Part model, mm, in its own coordinate system. Face numbers are marked on the shaded views. Round coordinates to 2 decimals unless told otherwise and drop trailing zeros. Write each loop counter-clockwise with the first axis right and the second up, starting at its lowest first coordinate (ties: lowest second). Pieces come first, ordered by that corner, then holes. Notation, with made-up numbers: M -10,14 L 9,14 A7 cw 9,27 Z; hole C 64,15 d6. An arc over 180 degrees is marked long. One line per question, with ' | ' between items. Start each with the question number.
1) Saw through at B-B (y = 31.75). List the corners of the cut face in (x, z) (3 decimals), plus the area to 3 significant figures.
2) Mould opens along Y. For the marked faces 1 and 2 say: pulls with the +Y half, pulls with the -Y half, needs draft (parallel to the pull), parting line crosses it, or undercut.
3) Drop flat-ended pins along their axis: pin 1 Ø9 at (x, y) = (-12.7, 19.05) entering from -Z; pin 2 Ø7 at (x, y) = (-12.7, 57.15) entering from +Z; pin 3 Ø6 at (x, y) = (10, -99.5) entering from -Z; pin 4 Ø12 at (y, z) = (-146, -101) entering from -X (3 decimals). Give the stop position or say it passes through.
4) Saw through at D-D (y = -106). List the corners of the cut face in (x, z) (3 decimals).
5) Saw through at C-C (z = -104.5). List the corners of the cut face in (x, y) (3 decimals), plus the area to 3 significant figures.
6) Saw through at A-A (x = -4). List the corners of the cut face in (y, z), plus the area to 3 significant figures.
7) Wall check: probe 1 along X at (y, z) = (44, -3) (3 decimals); probe 2 along Y at (x, z) = (0.5, -130.5); probe 3 along X at (y, z) = (81, -4) (3 decimals). Give the ranges that are in metal, low to high. Write a range as [from, to].
```python
from build123d import *

# Parameters (mm, degrees)
F0_W          = 49.53
F0_H          = 17.78
F3_DEPTH      = 127
F5_DEPTH      = 12.7
F5_DEPTH_BACK = 12.7
F6_R          = 3.81
F7_DEPTH      = 24.765
F7_DEPTH_BACK = 24.765
F8_R          = 6.35
F9_R          = 3.81
F10_DEPTH     = 6.35
F12_R         = 3.81
F13_DEPTH     = 25.4


with BuildPart() as f2:
    # F2: sweep along a path in F1
    with BuildLine(Plane.YZ) as f2_path:
        ThreePointArc((0, 0), (-117.5329964843, -42.794837435), (-177.8, -152.4))
    # F0 (on Front) → F2 (sweep)
    with BuildSketch(Plane.XZ):
        Rectangle(F0_W, F0_H)
    sweep(path=f2_path.line)

    # F0 (on Front) → F3 (join)
    with BuildSketch(Plane.XZ):
        Rectangle(F0_W, F0_H)
    extrude(amount=-F3_DEPTH)

    # F4 (on Right) → F5 (join, two sides)
    with BuildSketch(Plane.YZ) as f5_sk:
        Polygon((-169.126565554, -153.0713479475), (0, -7.7078141163), (-6.6193065428, 0), (-175.749050011, -145.3662652344), align=None)
    extrude(amount=F5_DEPTH)
    extrude(f5_sk.sketch, amount=-F5_DEPTH_BACK)

    # F8
    f8_edges = [f2.edges().sort_by_distance(p)[0] for p in [
        (0, -186.611435, -151.220714),
    ]]
    fillet(f8_edges, radius=F8_R)



with BuildPart() as f7:
    # F6 (on Right) → F7 (new body, two sides)
    with BuildSketch(Plane.YZ) as f7_sk:
        with Locations((-191.0524220981, -128.3607142857)):
            Circle(F6_R)
    extrude(amount=F7_DEPTH)
    extrude(f7_sk.sketch, amount=-F7_DEPTH_BACK)


with BuildPart() as f2_1:
    add(f2.part)

    add(f7.part)  # F10 merges F7
    # F9 (on face) → F10 (join)
    with BuildSketch(Plane(origin=(-24.765, 0, 0), x_dir=(0, -1, 0), z_dir=(-1, 0, 0))):
        with BuildLine():
            Line((186.7554907347, -139.1305014455), (193.8819702362, -136.7905924285))
            ThreePointArc((193.8819702362, -136.7905924285), (199.5987163414, -125.7076478809), (188.6094911041, -119.8127539412))
            Line((188.6094911041, -119.8127539412), (182.4592318073, -121.6144030093))
            ThreePointArc((182.4592318073, -121.6144030093), (180.5599939589, -121.4233791934), (179.3300967362, -119.9636027295))
            ThreePointArc((179.3300967362, -119.9636027295), (182.5296358067, -130.9094781954), (185.0548897469, -142.0302844844))
            ThreePointArc((185.0548897469, -142.0302844844), (185.3568434553, -140.2588106009), (186.7554907347, -139.1305014455))
        make_face()
        with Locations((191.10869103, -128.344230937)):
            Circle(F9_R, mode=Mode.SUBTRACT)
    extrude(amount=-F10_DEPTH)

    # F11: F2 across plane


with BuildPart() as f2_2:
    add(f2_1.part)
    add(f2_1.part.mirror(Plane.YZ))

    # F12 (on face) → F13 (cut)
    with BuildSketch(Plane.XY.offset(8.89)):
        with Locations((-12.7, 6.35)):
            Circle(F12_R)
        with Locations((-12.7, 19.05)):
            Circle(F12_R)
        with Locations((-12.7, 31.75)):
            Circle(F12_R)
        with Locations((-12.7, 44.45)):
            Circle(F12_R)
        with Locations((-12.7, 57.15)):
            Circle(F12_R)
        with Locations((-12.7, 69.85)):
            Circle(F12_R)
        with Locations((-12.7, 82.55)):
            Circle(F12_R)
        with Locations((-12.7, 95.25)):
            Circle(F12_R)
        with Locations((-12.7, 107.95)):
            Circle(F12_R)
        with Locations((-12.7, 120.65)):
            Circle(F12_R)
        with Locations((12.7, 6.35)):
            Circle(F12_R)
        with Locations((12.7, 19.05)):
            Circle(F12_R)
        with Locations((12.7, 31.75)):
            Circle(F12_R)
        with Locations((12.7, 44.45)):
            Circle(F12_R)
        with Locations((12.7, 57.15)):
            Circle(F12_R)
        with Locations((12.7, 69.85)):
            Circle(F12_R)
        with Locations((12.7, 82.55)):
            Circle(F12_R)
        with Locations((12.7, 95.25)):
            Circle(F12_R)
        with Locations((12.7, 107.95)):
            Circle(F12_R)
        with Locations((12.7, 120.65)):
            Circle(F12_R)
    extrude(amount=-F13_DEPTH, mode=Mode.SUBTRACT)


solid = f2_2.part
```
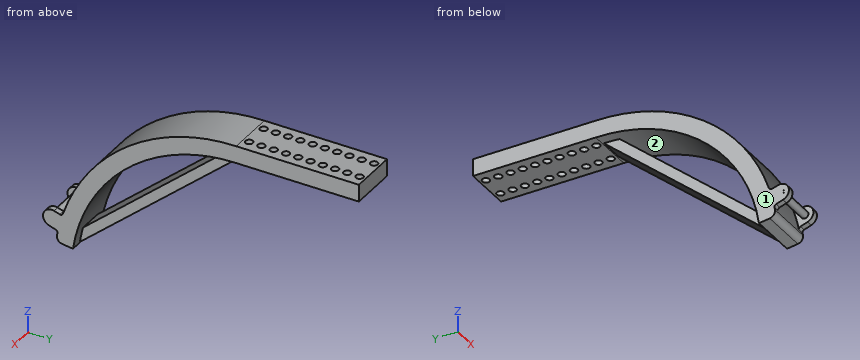
Answer key:
1) outline: M -24.765,-8.89 L -16.51,-8.89 L -16.51,8.89 L -24.765,8.89 Z; M -8.89,-8.89 L 8.89,-8.89 L 8.89,8.89 L -8.89,8.89 Z; M 16.51,-8.89 L 24.765,-8.89 L 24.765,8.89 L 16.51,8.89 Z | area: 610 mm2
2) face 1: needs draft | face 2: undercut
3) pin 1: stops at z = -8.89 | pin 2: passes through | pin 3: stops at z = -95.81 | pin 4: stops at x = -24.765
4) outline: M -24.765,-44.833 L 24.765,-44.833 L 24.765,-22.871 L -24.765,-22.871 Z; M -12.7,-98.814 L 12.7,-98.814 L 12.7,-85.417 L -12.7,-85.417 Z
5) outline: M -24.765,-173.524 L 24.765,-173.524 L 24.765,-154.004 L -24.765,-154.004 Z; M -12.7,-128.202 L 12.7,-128.202 L 12.7,-112.615 L -12.7,-112.615 Z | area: 1,360 mm2
6) outline: C -191.05,-128.36 d7.62; M -185.55,-144.67 A6.35 ccw -180.14,-152.09 L -168.99,-153.58 A168.91 cw -168.88,-152.86 L -1.36,-8.88 A168.91 cw 0,-8.89 L 127,-8.89 L 127,8.89 L 0,8.89 A186.69 ccw Z; hole M -165.66,-136.69 L -17.84,-9.64 A168.91 ccw Z | area: 8,960 mm2
7) probe 1: x = [-24.765, -16.483], [-8.917, 8.917], [16.483, 24.765] | probe 2: y = [-194.21, -187.9], [-182.42, -163.98], [-158.45, -142.87] | probe 3: x = [-24.765, -16.18], [-9.22, 9.22], [16.18, 24.765]
